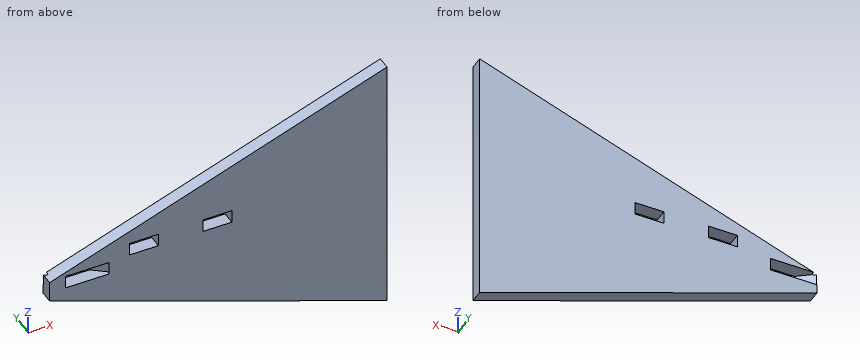
from build123d import *

# Parameters (mm, degrees)
BOX005_W               = 10
BOX005_H               = 154
BOX005_DEPTH           = 4.5
BOX005_PLACEMENT_ANGLE = 53
BOX001_W               = 10
BOX001_H               = 232
BOX001_DEPTH           = 4.5
BOX_W                  = 10
BOX_H                  = 232
BOX_DEPTH              = 4.5
PAD_DEPTH              = 4.5


with BuildPart() as left_front_spar:
    # Box005 → Box005 (new body)
    with BuildSketch(Plane.XY):
        with Locations((5, 77)):
            Rectangle(BOX005_W, BOX005_H)
    extrude(amount=BOX005_DEPTH)


with BuildPart() as left_front_spar_1:
    # Box005 placement: moved
    add(left_front_spar.part.moved(Location((152.246967, -91.722363, -2.4))).rotate(Axis((152.246967, -91.722363, -2.4), (0, 0, 1)), BOX005_PLACEMENT_ANGLE))


with BuildPart() as cube001:
    # Box001 → Box001 (new body)
    with BuildSketch(Plane(origin=(164.7, -92.4, 2.5), x_dir=(1, 0, 0), z_dir=(0, 0, 1))):
        with Locations((5, 116)):
            Rectangle(BOX001_W, BOX001_H)
    extrude(amount=BOX001_DEPTH)


with BuildPart() as cube:
    # Box → Box (new body)
    with BuildSketch(Plane(origin=(190, -89.9, 2.5), x_dir=(1, 0, 0), z_dir=(0, 0, 1))):
        with Locations((5, 116)):
            Rectangle(BOX_W, BOX_H)
    extrude(amount=BOX_DEPTH)


with BuildPart() as cut029:
    # Sketch → Pad (new body)
    with BuildSketch(Plane.XZ):
        Polygon((-112.766838, 5.66261), (-112.766838, -1.625728), (3.473136, -43.933619), (3.473136, 47.970501), align=None)
    extrude(amount=PAD_DEPTH)


with BuildPart() as cut029_1:
    # Body placement: moved
    add(cut029.part.moved(Location((250, -80, -4))))

    # Cut010: cut Cube
    add(cube.part, mode=Mode.SUBTRACT)

    # Cut022: cut Cube001
    add(cube001.part, mode=Mode.SUBTRACT)

    # Cut029: cut left front spar
    add(left_front_spar_1.part, mode=Mode.SUBTRACT)


solid = cut029_1.part
Design review of the part built by this model. Coordinates are the model's own, in mm. Give positions to 0.01 mm unless a question says otherwise; leave off trailing zeros. Loops run counter-clockwise (first coordinate to the right, second up) from the corner with the lowest first, then second, coordinate; pieces in that order, holes last. Notation, with made-up numbers: M 75,62 L 126,62 A21 cw 126,72 Z; hole C 33,68 d8. An arc over 180 degrees is marked long. Write item = value, one per line.
Q1. We need section A-A (x = 194). Give the boundary of the cut face in (y, z).
Output values:
outline = M -84.5,-26.29 L -80,-26.29 L -80,2.5 L -84.5,2.5 Z; M -84.5,7 L -80,7 L -80,22.32 L -84.5,22.32 Z
Q2. To check wall thickness, follow line 1 (Z direction, x = 147.5, y = -82.2); line 2 (Z direction, x = 146, y = -82.65); line 3 (X direction, y = -80.95, z = 0.5). State the ranges of each line that lie inside material, in increasing order. Write a range as [from, to].
Output values:
line_1 = [-9.36, -2.4], [2.1, 5.4]
line_2 = [-8.82, -2.4], [2.1, 4.85]
line_3 = [137.23, 137.95], [154.57, 253.47]
Q3. We need section B-B (y = -82.7). Give the boundary of the cut face in (x, z).
Output values:
outline = M 137.23,-5.63 L 253.47,-47.93 L 253.47,43.97 L 137.23,1.66 Z; hole M 140.27,-2.4 L 156.89,-2.4 L 156.89,2.1 L 140.27,2.1 Z; hole M 164.7,2.5 L 174.7,2.5 L 174.7,7 L 164.7,7 Z; hole M 190,2.5 L 200,2.5 L 200,7 L 190,7 Z
Q4. We need section D-D (x = 235). Give the boundary of the cut face in (y, z).
Output values:
outline = M -84.5,-41.21 L -80,-41.21 L -80,37.25 L -84.5,37.25 Z
Q5. Insertion check: pin 1 (1.3 mm diameter, centred on x = 196, y = -83.5, fed in from +Z); pin 2 (1 mm diameter, centred on x = 198, y = -81, fed in from -Z). Each pin has a flat end and moves straight along its axis. Give the tip position at first contact, or say it passes through.
Output values:
pin_1 = 23.29
pin_2 = -27.93
Q6. We need section C-C (z = 37). Give the boundary of the cut face in (x, y).
Output values:
outline = M 234.32,-84.5 L 253.47,-84.5 L 253.47,-80 L 234.32,-80 Z
